```python
from build123d import *

# Parameters (mm, degrees)
F1_DEPTH = 3.175
F2_R     = 12.7
F3_R     = 25.4


with BuildPart() as f1:
    # F0 (on Top) → F1 (new body)
    with BuildSketch(Plane.XY):
        with BuildLine():
            Line((9.035718, 92.67555), (21.014816, 79.365334))
            Line((21.014816, 79.365334), (45.719025, 101.598944))
            Line((45.719025, 101.598944), (45.719025, 139.698944))
            Line((45.719025, 139.698944), (12.699025, 139.698944))
            Line((12.699025, 139.698944), (12.699025, 101.757354))
            ThreePointArc((12.699025, 101.757354), (11.777927, 96.849164), (9.035718, 92.67555))
        make_face()
        with BuildLine():
            ThreePointArc((0, 0), (4.86008, -0.96673), (8.980256, -3.719744))
            Line((8.980256, -3.719744), (20.956198, 9.587422))
            Line((20.956198, 9.587422), (-17.780975, 44.449402))
            Line((-17.780975, 44.449402), (21.014816, 79.365334))
            Line((21.014816, 79.365334), (9.035718, 92.67555))
            ThreePointArc((9.035718, 92.67555), (4.896401, 89.881841), (0, 88.9))
            Line((0, 88.9), (0, 81.28))
            Line((0, 81.28), (-78.74, 81.28))
            Line((-78.74, 81.28), (-78.74, 68.58))
            Line((-78.74, 68.58), (-78.74, 7.62))
            Line((-78.74, 7.62), (0, 7.62))
            Line((0, 7.62), (0, 0))
        make_face()
        with BuildLine():
            ThreePointArc((8.980256, -3.719744), (11.73327, -7.83992), (12.7, -12.7))
            Line((12.7, -12.7), (12.7, -50.8))
            Line((12.7, -50.8), (45.72, -50.8))
            Line((45.72, -50.8), (45.72, -12.699057))
            Line((45.72, -12.699057), (20.956198, 9.587422))
            Line((20.956198, 9.587422), (8.980256, -3.719744))
        make_face()
        Polygon((-88.9, 7.62), (-78.74, 7.62), (-78.74, 68.58), (-78.74, 81.28), (-88.9, 81.28), (-88.9, 88.9), (-114.3, 69.85), (-114.3, 19.05), (-88.9, 0), align=None)
    extrude(amount=F1_DEPTH)

    # F2
    f2_edges = [f1.edges().sort_by_distance(p)[0] for p in [
        (-114.3, 69.85, 1.5875),
        (-114.3, 19.05, 1.5875),
        (12.7, -50.8, 1.5875),
        (45.72, -50.8, 1.5875),
        (45.719025, 139.698944, 1.5875),
        (12.699025, 139.698944, 1.5875),
    ]]
    fillet(f2_edges, radius=F2_R)

    # F3
    f3_edges = [f1.edges().sort_by_distance(p)[0] for p in [
        (45.719025, 101.598944, 1.5875),
        (45.72, -12.699057, 1.5875),
    ]]
    fillet(f3_edges, radius=F3_R)


solid = f1.part
```
Build history of the part. All positions in model axes, mm. A direction names the side the tool comes from. Give positions to 0.01 mm unless a question says otherwise; leave off trailing zeros. Loops run counter-clockwise (first coordinate to the right, second up) from the corner with the lowest first, then second, coordinate; pieces in that order, holes last.
1) 3-axis set-ups, long thin cutter, end or side, ignore diameter. For faces 4 (the face through (41.9, -47.18, 1.61)), 5 (the face through (43.46, -13.54, 1.61)): which of +Z, -Z, +X, -X, +Y, -Y reach the whole face in a straight line?
Values follow:
face 4: +Z, -Z, +X, -Y
face 5: +Z, -Z, +X
2) Band-saw the part on C-C on x = -22. List the corners of the cut face in (y, z) (3 decimals).
Values follow:
outline: (7.62, 0) - (81.28, 0) - (81.28, 3.175) - (7.62, 3.175) - close
3) Two-plate mould, pull along Y, no slides. Class faces 1 (the face through (43.58, 102.71, 1.61)), 2 (the face through (42.1, 135.88, 1.61)), 3 (the face through (-99.202, 7.727, 1.565)): released by +Y, released by -Y, zero draft, split by the parting line, or undercut.
Values follow:
face 1: undercut
face 2: released by +Y
face 3: released by -Y
4) Probe line 1 along Y through (x, z) = (-63, 2.25); line 2 along X through (y, z) = (125, 0.2); line 3 along X through (y, z) = (88, 0.45). List the from-to ranges inside material, lowest first.
Values follow:
line 1: y = 7.62 to 81.28
line 2: x = 12.7 to 45.72
line 3: x = -90.1 to -88.9, 0 to 30.61
5) Band-saw the part on B-B on y = 115.5. List the corners of the cut face in (x, z) (3 decimals).
Values follow:
outline: (12.699, 0) - (45.719, 0) - (45.719, 3.175) - (12.699, 3.175) - close
6) Drop flat-ended pins along their axis: P1, Ø1, axis at x = -30.5, z = 2, coming from the -Y side; P2, Ø1, axis at y = 110.5, z = 2, coming from the -X side; P3, Ø1, axis at y = 84.5, z = 2, coming from the +X side. Give the stop position or say it passes through.
Values follow:
P1: stops at y = 7.62
P2: stops at x = 12.7
P3: stops at x = 27.28
